```python
from build123d import *

# Parameters (mm, degrees)
F0_W      = 1260
F0_H      = 1230
F1_DEPTH  = 1990
F3_DEPTH  = 25
F4_DEPTH  = 25
F5_W      = 919.1210865974
F5_H      = 1030.3928852081
F6_DEPTH  = 3660
F7_DEPTH  = 25
F8_W      = 712.8995805979
F8_H      = 942.8355097771
F9_DEPTH  = 3440
F10_W     = 919.1210865974
F10_H     = 347.6484620571
F11_DEPTH = 350
F11_TAPER = 25


with BuildPart() as f1:
    # F0 (on Top) → F1 (new body)
    with BuildSketch(Plane.XY):
        Rectangle(F0_W, F0_H)
    extrude(amount=F1_DEPTH)

    # F2 (on face) → F3 (cut)
    with BuildSketch(Plane(origin=(0, 615, 0), x_dir=(-1, 0, 0), z_dir=(0, 1, 0))):
        with BuildLine():
            add(Edge.make_bspline(
                [(-233.063429594, 1101.6209125519), (-392.2844546987, 1101.6209125519), (-312.6739421464, 887.6741528511), (-233.063429594, 673.7273931503), (-153.4529170417, 887.6741528511), (-73.8424044893, 1101.6209125519), (-233.063429594, 1101.6209125519)],
                knots=[0, 0, 0, 2.0943951024, 2.0943951024, 4.1887902048, 4.1887902048, 6.2831853072, 6.2831853072, 6.2831853072], degree=2, weights=[1, 0.5, 1, 0.5, 1, 0.5, 1]))
        make_face()
        with BuildLine():
            add(Edge.make_bspline(
                [(225.3940701485, 1111.8088960648), (65.7797781257, 1111.8088960648), (145.5869241371, 882.5801610947), (225.3940701485, 653.3514261246), (305.2012161599, 882.5801610947), (385.0083621713, 1111.8088960648), (225.3940701485, 1111.8088960648)],
                knots=[0, 0, 0, 2.0943951024, 2.0943951024, 4.1887902048, 4.1887902048, 6.2831853072, 6.2831853072, 6.2831853072], degree=2, weights=[1, 0.5, 1, 0.5, 1, 0.5, 1]))
        make_face()
        with BuildLine():
            Line((-338.4010910988, 1285.003900528), (338.4010910988, 1285.003900528))
            ThreePointArc((338.4010910988, 1285.003900528), (373.7564301581, 1299.6485614686), (388.4010910988, 1335.003900528))
            Line((388.4010910988, 1335.003900528), (388.4010910988, 1744.4011688232))
            ThreePointArc((388.4010910988, 1744.4011688232), (373.7564301581, 1779.7565078826), (338.4010910988, 1794.4011688232))
            Line((338.4010910988, 1794.4011688232), (-338.4010910988, 1794.4011688232))
            ThreePointArc((-338.4010910988, 1794.4011688232), (-373.7564301581, 1779.7565078826), (-388.4010910988, 1744.4011688232))
            Line((-388.4010910988, 1744.4011688232), (-388.4010910988, 1335.003900528))
            ThreePointArc((-388.4010910988, 1335.003900528), (-373.7564301581, 1299.6485614686), (-338.4010910988, 1285.003900528))
        make_face()
    extrude(amount=-F3_DEPTH, mode=Mode.SUBTRACT)

    # F4 (add): a face of the model
    f4_faces = [f1.faces().sort_by_distance(p)[0] for p in [
        (0.1841211697, 615, 890.8357911974),
    ]]
    extrude(f4_faces, amount=F4_DEPTH)

    # F5 (on face) → F6 (cut)
    with BuildSketch(Plane(origin=(0, 640, 0), x_dir=(-1, 0, 0), z_dir=(0, 1, 0))):
        Rectangle(F5_W, F5_H)
    extrude(amount=-F6_DEPTH, mode=Mode.SUBTRACT)

    # F7 (add): a face of the model
    f7_faces = [f1.faces().sort_by_distance(p)[0] for p in [
        (630, 12.5, 995),
    ]]
    extrude(f7_faces, amount=F7_DEPTH)

    # F8 (on face) → F9 (cut)
    with BuildSketch(Plane.YZ.offset(655)):
        with Locations((88.3218422532, 0)):
            Rectangle(F8_W, F8_H)
    extrude(amount=-F9_DEPTH, mode=Mode.SUBTRACT)

    # F10 (on face) → F11 (join)
    with BuildSketch(Plane(origin=(0, 0, 515.1964426041), x_dir=(1, 0, 0), z_dir=(0, 0, -1))):
        with Locations((0, 441.1757689714)):
            Rectangle(F10_W, F10_H)
    extrude(amount=F11_DEPTH, taper=F11_TAPER)


solid = f1.part
```
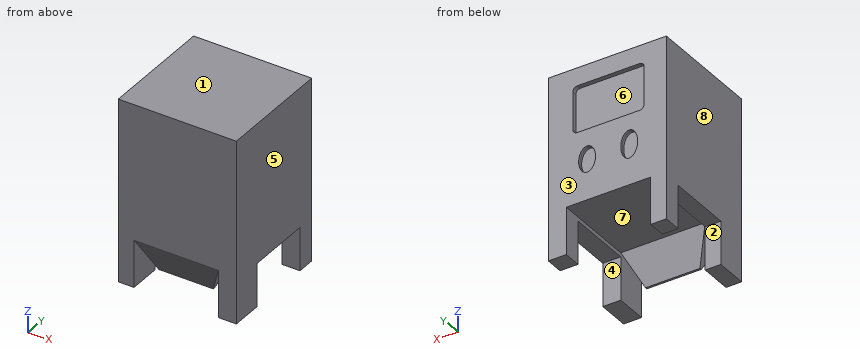
The listing builds one solid part. Answer for the finished solid, in the listing's coordinates (mm). Face numbers are marked on the shaded views. A direction names the side the tool comes from. Coordinates: 2 decimals unless noted, no trailing zeros. Write each loop counter-clockwise with the first axis right and the second up, starting at its lowest first coordinate (ties: lowest second). Pieces come first, ordered by that corner, then holes. Notation, with made-up numbers: M -20.75,84 L 13.25,84 A14 cw 13.25,103 Z; hole C 81.25,30.5 d1. An arc over 180 degrees is marked long. Use a Markdown table: item, result. Add a question column.
1. Given P1, Ø12, axis at x = 297.5, y = -283.5, coming from the -Z side; P2, Ø25, axis at x = 21.5, y = 624.5, coming from the -Z side; P3, Ø17, axis at x = 61, y = -441.5, coming from the -Z side, each flat-ended and moving along its own axis, determine where each tip first touches the part or whether it passes through.
2. For a pull along Y with two mould halves and no side action, classify the marked faces 1, 2 and 3 as +Y half, -Y half, draft (parallel to the pull), parting line (faces both ways), or undercut.
3. Which of the six approach directions +Z, -Z, +X, -X, +Y, -Y give full straight-line access (tool end or side, diameter ignored) to the marked faces 4, 5, 6, 7 and 8?
4. Straight lines are drawn through the part: line 1 along Y through (x, z) = (495, 409); line 2 along X through (y, z) = (-442, 350.5); line 3 along Y through (x, z) = (284.5, 1715). For each, find the intervals that lie inside material, in ascending order. Write a range as [from, to].
5. Section A-A (z = 1595) is taken. Give the vertices of the cut face in (x, y), plus the area to 3 significant figures.
6. Section C-C (z = 380) is taken. Count the separate pieces of the cut face and the enclosed holes in it, plus the area to 3 significant figures.
7. Section B-B (y = 560) is taken. Give the vertices of the cut face in (x, z).
Data:
| question | item | result |
|---|---|---|
| 1 | P1 | stops at z = 467.7 |
| 1 | P2 | stops at z = 515.2 |
| 1 | P3 | stops at z = 165.2 |
| 2 | face 1 | draft |
| 2 | face 2 | undercut |
| 2 | face 3 | +Y half |
| 3 | face 4 | -Z, +X, -X |
| 3 | face 5 | +Z, -Z, +X, +Y, -Y |
| 3 | face 6 | +Y |
| 3 | face 7 | -Z, +Y |
| 3 | face 8 | +Z, -Z, -X, +Y, -Y |
| 4 | line 1 | y = [-615, -268.13], [444.77, 640] |
| 4 | line 2 | x = [-630, -459.56], [-382.76, 382.76], [459.56, 655] |
| 4 | line 3 | y = [-615, 590] |
| 5 | outline | M -630,-615 L 655,-615 L 655,640 L 388.4,640 L 388.4,590 L -388.4,590 L -388.4,640 L -630,640 Z |
| 5 | area | 1,570,000 mm2 |
| 6 | separate pieces | 5 |
| 6 | enclosed holes | 0 |
| 6 | area | 374,000 mm2 |
| 7 | outline | M -630,0 L -459.56,0 L -459.56,515.2 L 459.56,515.2 L 459.56,0 L 655,0 L 655,1990 L -630,1990 Z |
